Autodesk Inventor part; units mm, degrees
ref_plane "YZ Plane" through (0, 0, 0) normal (1, 0, 0) x (0, 1, 0)
ref_plane "XZ Plane" through (0, 0, 0) normal (0, 1, 0) x (-1, 0, 0)
ref_plane "XY Plane" through (0, 0, 0) normal (0, 0, 1) x (1, 0, 0)
sketch "Эскиз1" plane through (0, 0, 0) normal (0, 0, 1) x (1, 0, 0)
  line L0 (0, 0) -> (5.1, 0)
  line L1 (5.1, 0) -> (5.1, 6.8)
  line L2 (5.1, 6.8) -> (0, 6.8)
  line L3 (0, 6.8) -> (0, 0)
  line L4 (8.5, 0) -> (13.6, 0)
  line L5 (13.6, 0) -> (13.6, 6.8)
  line L6 (13.6, 6.8) -> (8.5, 6.8)
  line L7 (8.5, 6.8) -> (8.5, 0)
  line L8 (17, 0) -> (22.1, 0)
  line L9 (22.1, 0) -> (22.1, 6.8)
  line L10 (22.1, 6.8) -> (17, 6.8)
  line L11 (17, 6.8) -> (17, 0)
  line L12 (25.5, 0) -> (30.6, 0)
  line L13 (30.6, 0) -> (30.6, 6.8)
  line L14 (30.6, 6.8) -> (25.5, 6.8)
  line L15 (25.5, 6.8) -> (25.5, 0)
  line L16 (5.1, 6.8) -> (8.5, 6.8)
  line L17 (13.6, 6.8) -> (17, 6.8)
  line L18 (22.1, 6.8) -> (25.5, 6.8)
  line L19 (22.1, 5.4) -> (25.5, 5.4)
  line L20 (17, 5.4) -> (13.6, 5.4)
  line L21 (8.5, 5.4) -> (5.1, 5.4)
  line L22 (0, 5.4) -> (-1.6, 5.4)
  line L23 (-1.6, 5.4) -> (-1.6, 6.8)
  line L24 (-1.6, 6.8) -> (0, 6.8)
  line L25 (0, 6.8) -> (0, 5.4)
  line L26 (30.6, 5.4) -> (32.2, 5.4)
  line L27 (32.2, 5.4) -> (32.2, 6.8)
  line L28 (32.2, 6.8) -> (30.6, 6.8)
  line L29 (30.6, 6.8) -> (30.6, 5.4)
  dimension "d0" = 5.1
  dimension "d1" = 6.8
  dimension "d4" = 8.5
  dimension "d9" = 1.4
  dimension "d10" = 1.6
extrude "Выдавливание1" add sketch "Эскиз1" along normal blind 0.6
sketch "Эскиз2" plane through (0, 0, 0.6) normal (0, 0, 1) x (1, 0, 0)
  line L0 (0, 5.4) -> (0, 0)
  line L1 (5.1, 0) -> (5.1, 5.4)
  line L2 (0, 1.2) -> (5.1, 1.2)
  line L3 (5.1, 1.2) -> (5.1, 6.6)
  line L4 (5.1, 6.6) -> (0, 6.6)
  line L5 (0, 6.6) -> (0, 1.2)
  line L6 (8.5, 5.4) -> (8.5, 0)
  line L7 (13.6, 0) -> (13.6, 5.4)
  line L8 (8.5, 1.2) -> (13.6, 1.2)
  line L9 (13.6, 1.2) -> (13.6, 6.6)
  line L10 (13.6, 6.6) -> (8.5, 6.6)
  line L11 (8.5, 6.6) -> (8.5, 1.2)
  line L12 (17, 5.4) -> (17, 0)
  line L13 (22.1, 0) -> (22.1, 5.4)
  line L14 (17, 1.2) -> (22.1, 1.2)
  line L15 (22.1, 1.2) -> (22.1, 6.6)
  line L16 (22.1, 6.6) -> (17, 6.6)
  line L17 (17, 6.6) -> (17, 1.2)
  line L18 (25.5, 5.4) -> (25.5, 0)
  line L19 (30.6, 0) -> (30.6, 5.4)
  line L20 (25.5, 1.2) -> (30.6, 1.2)
  line L21 (30.6, 1.2) -> (30.6, 6.6)
  line L22 (30.6, 6.6) -> (25.5, 6.6)
  line L23 (25.5, 6.6) -> (25.5, 1.2)
  line L24 (0, 0) -> (5.1, 0)
  line L25 (32.2, 6.8) -> (-1.6, 6.8)
  point P0 (25.5, 5.5)
  point P1 (30.6, 1.2)
  point P2 (17, 5.5)
  point P3 (8.5, 5.5)
  point P4 (0, 5.5)
  dimension "d14" = 5.4
  dimension "d21" = 0.2
extrude "Выдавливание2" add sketch "Эскиз2" along normal blind 2.2 contours L5 L4 L3 L1 L2 L0 | L11 L10 L9 L7 L8 L6 | L17 L16 L15 L13 L14 L12 | L23 L22 L21 L19 L20 L18
sketch "Эскиз3" plane through (0, 0, 0) normal (-1, 0, 0) x (0, 0, 1)
  line L0 (0.6, 1.2) -> (2.8, 1.9)
  line L1 (0, 5.4) -> (0, 0)
  line L2 (0, 0) -> (0.6, 0)
  line L3 (0.6, 1.2) -> (0.6, 0)
  line L4 (0.6, 1.2) -> (2.8, 1.2)
  line L5 (2.8, 6.6) -> (2.8, 1.2)
  line L6 (0.6, 5.4) -> (0.6, 6.6)
  line L7 (0, 5.4) -> (0.6, 5.4)
  line L8 (0.6, 1.2) -> (2.8, 1.2)
  line L9 (0.6, 6.6) -> (2.8, 6.6)
  line L10 (0.6, 6.6) -> (2.8, 5.9)
  line L11 (2.8, 1.2) -> (2.8, 6.6)
  line L12 (2.8, 1.9) -> (2.8, 1.2)
  line L13 (0.6, 6.6) -> (2.8, 6.6)
  line L14 (0.6, 6.8) -> (0.6, 5.4)
  line L15 (2.8, 6.6) -> (2.8, 1.2)
  line L16 (2.8, 5.9) -> (2.8, 6.6)
  point P0 (2.8, 1.9)
  point P1 (2, 5.8)
  point P2 (2, 5.6739)
  point P3 (2, 5.8)
  dimension "d18" = 4
extrude "Выдавливание3" cut sketch "Эскиз3" against normal through all contours L0 L5 L4 | L10 L9 L5
properties part number "Buttons"
Read the model definition and answer for the solid it produces. Units are mm, in the model's axes. A direction names the side the tool comes from. Give positions to 0.01 mm unless a question says otherwise; leave off trailing zeros. Order: outer loops, then holes, each group sorted by start corner. A loop starts at its lowest first (then second) coordinate and runs counter-clockwise, first axis right, second up.
(1) Find section C-C (x = 13). Give the vertices of the cut face in (y, z), plus the area to 3 significant figures.
(2) Find section A-A (y = 3.5). Give the vertices of the cut face in (x, z).
(3) For faces 3 (the flat face through (15, 6, 0.6)), 4 (the flat face through (20, 1, 0.6)), 5 (the flat face through (13.6, 3, 1)), determine the directions among +Z, -Z, +X, -X, +Y, -Y from which every point of the face is accessible in a straight line to the end or side of a thin tool.
(4) Straight lines are drawn through the part: L1, parallel to X at y = 2.75, z = 1.2; L2, parallel to Z at x = 13, y = 0.75; L3, parallel to Y at x = 21, z = 1.6. For each, find the intervals that lie inside material, in ascending order.
(5) Given pin 1 (0.5 mm diameter, centred on x = -1, z = 0.5, fed in from -Y); pin 2 (1 mm diameter, centred on x = 29, y = 0.5, fed in from +Z); pin 3 (1.4 mm diameter, centred on y = 2, z = 2, fed in from +X), each flat-ended and moving along its own axis, determine where each tip first touches the part or whether it passes through.
(6) For a pull along X with two mould halves and no side action, classify faces 1 (the flat face through (28, 1, 0.6)), 2 (the flat face through (5.1, 3, 1)) as released by +X, released by -X, zero draft, split by the parting line, or undercut.
(7) Find section B-B (z = 1.7). Give the vertices of the cut face in (x, y), plus the area to 3 significant figures.
(8) Find section D-D (y = 6.25). Give the vertices of the cut face in (x, z), plus the area to 3 significant figures.
Result sheet:
1. outline: (0, 0) - (6.8, 0) - (6.8, 0.6) - (6.6, 0.6) - (5.9, 2.8) - (1.9, 2.8) - (1.2, 0.6) - (0, 0.6) - close
1. area: 14.4 mm2
2. outline: (0, 0) - (5.1, 0) - (5.1, 2.8) - (0, 2.8) - close; (8.5, 0) - (13.6, 0) - (13.6, 2.8) - (8.5, 2.8) - close; (17, 0) - (22.1, 0) - (22.1, 2.8) - (17, 2.8) - close; (25.5, 0) - (30.6, 0) - (30.6, 2.8) - (25.5, 2.8) - close
3. face 3: +Z, +Y
3. face 4: +Z, +X, -X, -Y
3. face 5: +Z, -Y
4. L1: x = 0 to 5.1, 8.5 to 13.6, 17 to 22.1, 25.5 to 30.6
4. L2: z = 0 to 0.6
4. L3: y = 1.52 to 6.28
5. pin 1: stops at y = 5.4
5. pin 2: stops at z = 0.6
5. pin 3: stops at x = 30.6
6. face 1: zero draft
6. face 2: undercut
7. outline: (0, 1.55) - (5.1, 1.55) - (5.1, 6.25) - (0, 6.25) - close; (8.5, 1.55) - (13.6, 1.55) - (13.6, 6.25) - (8.5, 6.25) - close; (17, 1.55) - (22.1, 1.55) - (22.1, 6.25) - (17, 6.25) - close; (25.5, 1.55) - (30.6, 1.55) - (30.6, 6.25) - (25.5, 6.25) - close
7. area: 95.9 mm2
8. outline: (-1.6, 0) - (32.2, 0) - (32.2, 0.6) - (30.6, 0.6) - (30.6, 1.7) - (25.5, 1.7) - (25.5, 0.6) - (22.1, 0.6) - (22.1, 1.7) - (17, 1.7) - (17, 0.6) - (13.6, 0.6) - (13.6, 1.7) - (8.5, 1.7) - (8.5, 0.6) - (5.1, 0.6) - (5.1, 1.7) - (0, 1.7) - (0, 0.6) - (-1.6, 0.6) - close
8. area: 42.7 mm2
